Check sheet for the modelled part. Datum: model origin and axes. Units: mm. A direction names the side the tool comes from. Round coordinates to 2 decimals unless told otherwise and drop trailing zeros. Loops run counter-clockwise (first coordinate to the right, second up) from the corner with the lowest first, then second, coordinate; pieces in that order, holes last. Notation, with made-up numbers: (35, -14) -> (91, -14) arc R25 ccw to (91, 3) -> close; hole circle Ø4 at (14, 11). An arc over 180 degrees is marked (long way). One line per question, with ' | ' between items.
Autodesk Inventor part; units mm, degrees
sketch "HeadplateSketch" plane through (0, 0, 0) normal (0, 0, 1) x (1, 0, 0)
  line L0 (22.2193, -2.4109) -> (25.4193, -1.6109)
  line L1 (25.4193, -1.6109) -> (25.4193, -0.0109)
  line L2 (6.3193, 0.7891) -> (3.1193, -0.0109)
  line L3 (3.1193, -1.6109) -> (3.1193, -0.0109)
  line L4 (6.3193, 0.7891) -> (22.2193, 0.7891)
  line L5 (22.2193, 0.7891) -> (25.4193, -0.0109)
  line L6 (17.1922, 9.6958) -> (17.1922, -2.4109)
  line L7 (17.1922, 9.6958) -> (18.128, 9.6958)
  line L8 (17.1922, 9.6958) -> (15.1602, 9.6958)
  line L9 (11.7996, 5.443) -> (11.7996, -2.4109)
  line L10 (21.4383, 5.5008) -> (21.4383, -2.4109)
  line L11 (21.4383, 5.5008) -> (18.128, 9.6958)
  arc A0 (15.1602, 9.6958) -> (11.7996, 5.443) centre (17.4689, 4.4173) ccw
  line L12 (3.1193, -1.6109) -> (6.3193, -2.4109)
  line L13 (6.3193, -2.4109) -> (22.2193, -2.4109)
  point P0 (11.7996, 0.7891)
  dimension "d95" = 3.2
  dimension "d102" = 1.6
  dimension "d104" = 3.2
  dimension "d106" = 0.8
  dimension "d109" = 1.6
  dimension "d110" = 3.2
  dimension "d112" = 22.3
  dimension "d113" = 15.9
extrude "拉伸1" add sketch "HeadplateSketch" along normal blind 1.27
extrude "拉伸8" add sketch "HeadplateSketch" against normal blind 1.5 contours L13 L6 L4 L10 | L4 L6 L7 L11 L10 | L13 L9 L4 L6 | L4 L9 A0 L8 L6
sketch "草图2" plane through (15.1602, 9.6958, 1.27) normal (0, 1, 0) x (1, 0, 0)
  line L0 (-3.3633, 2.0352) -> (1.9994, 0)
  arc A0 (-3.3633, 2.77) -> (6.2787, 1.2693) centre (3.7754, 16.9113) ccw
  line L1 (1.9994, 0) -> (6.2787, 0)
  line L2 (-3.3633, 2.77) -> (6.2787, 2.77)
  line L3 (2.9678, 2.77) -> (0, 2.77)
  line L4 (6.2787, 1.2693) -> (6.2787, 2.77)
  line L5 (-3.3633, 0) -> (1.9994, 0)
  line L6 (0, 0) -> (2.9678, 0)
  line L7 (2.9678, 0) -> (2.9678, 2.77)
  line L8 (-3.3633, 0) -> (-3.3633, 2.0352)
extrude "拉伸4" cut sketch "草图2" against normal up to next contours A0 L2 L7 | L7 L2 L4 A0
sketch "草图6" plane through (6.3193, -2.4109, 0) normal (0, -1, 0) x (1, 0, 0)
  line L0 (0, 0) -> (5.5435, 0)
  line L1 (0.6566, 0) -> (5.5435, -1.4987)
  line L2 (5.5435, 0) -> (5.5435, -1.4987)
  line L3 (0.6566, 0) -> (5.5435, 0)
  arc A0 (15.1197, 0.0007) -> (5.4803, -1.4987) centre (12.6164, -15.6413) ccw
  line L4 (15.1197, 0.0007) -> (15.1197, 0)
  line L5 (15.1197, 0) -> (15.9, 0)
  line L6 (15.9, 0) -> (15.9, 1.27)
  line L7 (15.9, 1.27) -> (0, 1.27)
  line L8 (0, 0) -> (0, 1.27)
  line L9 (0, 0) -> (5.4803, 0)
  line L10 (5.4803, 0) -> (5.4803, -1.4987)
extrude "拉伸7" add sketch "草图6" against normal up to surface (3.2 mm away) contours L0 L10 L1 | L0 L2 A0 L1 L10 | A0 L2 L1
sketch "草图3" plane through (6.3193, 0.7891, 0) normal (0, 1, 0) x (1, 0, 0)
  line L0 (0, -1.27) -> (5.4803, -1.27)
  line L1 (5.4803, 0) -> (5.4803, -1.27)
  line L2 (5.4803, 0) -> (0, 0)
  line L3 (0, 0) -> (0, -1.27)
  line L4 (5.4803, -1.27) -> (16.1538, -1.27)
  line L5 (16.1538, -1.27) -> (17.1139, -1.27)
  line L6 (17.1139, -1.27) -> (17.1139, 0.0011)
extrude "拉伸9" cut sketch "草图2" against normal up to surface (8.9067 mm away) contours L0 L5 L8
sketch "草图4" plane through (0, 0, 1.27) normal (0, 0, 1) x (1, 0, 0)
  circle A0 centre (17.2686, 8.053) radius 0.825
  circle A1 centre (18.9292, 5.4282) radius 0.825
  circle A2 centre (19.0006, 2.5892) radius 0.825
  circle A3 centre (17.1095, -0.097) radius 0.825
  line L0 (6.3193, 0.7891) -> (11.7996, 0.7891)
  line L1 (12.1356, 5.3815) -> (12.1356, 2.0023)
  line L2 (12.1356, 5.3815) -> (17.1561, 5.3815)
  line L3 (17.1561, 5.3815) -> (17.1561, 2.008)
  line L4 (17.1561, 2.008) -> (12.1356, 2.008)
  line L5 (11.7983, 4.0675) -> (12.1356, 4.0675)
  arc A4 (17.1561, 5.3815) -> (12.1356, 5.3815) centre (14.6459, 4.9584) ccw
  arc A5 (12.1356, 2.008) -> (17.1561, 2.008) centre (14.6459, 5.3033) ccw
  circle A6 centre (19.9896, -0.0785) radius 0.825
  circle A7 centre (14.1001, -0.1524) radius 0.825
extrude "拉伸10" cut sketch "草图4" against normal through all contours L2 L3 L4 L1 | A4 L2 | L4 A5
hole "打孔7" at (18.9292, 5.4282, 1.27) at (19.0006, 2.5892, 1.27) at (17.1095, -0.097, 1.27) at (17.2686, 8.053, 1.27) direction (0, 0, -1) diameter 1.65 end through all
hole "打孔8" at (14.1001, -0.1524, 1.27) at (19.9896, -0.0785, 1.27) direction (0, 0, -1) diameter 1.65 end through all
sketch "Sketch8" plane through (0, 0, 0) normal (0, 0, 1) x (1, 0, 0)
  arc A0 (17.1561, 5.3815) -> (12.1356, 5.3815) centre (14.6459, 4.9584) ccw
  arc A1 (12.1356, 2.008) -> (17.1561, 2.008) centre (14.6459, 5.3033) ccw
  line L0 (17.1596, 7.2353) -> (17.1596, 0.7891)
  line L1 (12.1356, 2.008) -> (12.1356, 5.3815)
  line L2 (14.6459, 7.5041) -> (14.6459, 1.1608)
  line L3 (17.1596, 4.3324) -> (12.1356, 4.3324)
  line L4 (-5.0839, 0) -> (30.5031, 0)
  line L5 (0, 12.1209) -> (0, -4.8328)
  point P0 (0, 0)
  dimension "d116" = 6.3433
  dimension "d117" = 3.1717
  dimension "d118" = 14.6459
  dimension "d119" = 4.3324
sketch "Sketch9" plane through (11.7996, 0.7891, -0.7642) normal (-0.3548, 0, 0.9349) x (0.9349, 0, 0.3548)
  ellipse E0 centre (5.8496, 7.2639) end of major axis (6.7321, 7.2639) minor radius 0.825 (5.7331, 8.0816) -> (5.7331, 6.4461) ccw
  line L0 (5.7331, 8.9067) -> (5.7331, 8.0816)
  line L1 (3.5945, 8.9067) -> (5.7331, 8.9067)
  ellipse E1 centre (6.0638, 3.6282) end of major axis (-0.0984, 3.6282) minor radius 5.7613 (3.5945, 8.9067) -> (0, 4.6539) ccw
  line L2 (0, 0) -> (0, 4.6539)
  line L3 (0, 0) -> (5.7331, 0)
  line L4 (5.7331, 6.4461) -> (5.7331, 0)
  line L5 (5.7293, 4.5923) -> (5.7293, 1.2188)
  ellipse E2 centre (3.0444, 4.5141) end of major axis (-1.3864, 4.5141) minor radius 4.1425 (0.3594, 1.2188) -> (5.7293, 1.2188) ccw
  line L6 (0.3594, 1.2188) -> (0.3594, 4.5923)
  ellipse E3 centre (3.0444, 4.1693) end of major axis (5.7672, 4.1693) minor radius 2.5457 (5.7293, 4.5923) -> (0.3594, 4.5923) ccw
  line L7 (5.3145, 1.2188) -> (5.3145, 4.5923)
  arc A0 (0.112, 1.2188) -> (5.3145, 1.2188) centre (5.3145, 1.2188) ccw
  arc A1 (5.3145, 4.5923) -> (0.112, 4.5923) centre (0.112, 4.5923) ccw
  line L8 (5.3145, 4.5923) -> (0.3594, 4.5923)
  line L9 (2.8369, 6.7075) -> (4.6638, 6.7075)
  line L10 (2.8369, 0.3762) -> (5.3145, 0.3762)
  line L11 (2.8369, 6.7075) -> (2.8369, 0.3762)
  line L12 (2.8369, 3.5419) -> (5.3145, 3.5419)
  line L13 (2.9322, 6.7149) -> (2.9322, 0.3716)
  point P0 (-10.7607, -0.7891)
  dimension "d121" = 0.0953
ref_plane "Work Plane3" through (11.7996, 0.7891, -0.7642) normal (-0.3548, 0, 0.9349) x (0.9349, 0, 0.3548)
ref_plane "Work Plane1" through (14.558, 0, 0) normal (1, 0, 0) x (0, 1, 0)
ref_plane "Work Plane2" through (0, 4.332, 0) normal (0, 1, 0) x (-1, 0, 0)
ref_plane "Work Plane4" through (0, 0, 0.283) normal (0, 0, 1) x (1, 0, 0)
sketch "Sketch10" plane through (0, 0, 0) normal (0, 0, 1) x (1, 0, 0)
  line L0 (3.1193, -1.6109) -> (3.1193, -0.0109)
  line L1 (3.1193, -0.8109) -> (0, -0.8109)
  line L2 (25.404, -0.8109) -> (34.4809, -0.8109)
  point P0 (0, 0)
  dimension "d126" = 0.8109
ref_plane "Work Plane5" through (0, -0.811, 0) normal (0, 1, 0) x (-1, 0, 0)
sketch "Sketch11" plane through (11.7996, 0.7891, -0.7642) normal (-0.3548, 0, 0.9349) x (0.9349, 0, 0.3548)
  ellipse E0 centre (5.8496, 7.2639) end of major axis (6.7321, 7.2639) minor radius 0.825 (5.7331, 8.0816) -> (5.7331, 6.4461) ccw
  line L0 (5.7331, 8.9067) -> (5.7331, 8.0816)
  line L1 (3.5945, 8.9067) -> (5.7331, 8.9067)
  ellipse E1 centre (6.0638, 3.6282) end of major axis (-0.0984, 3.6282) minor radius 5.7613 (3.5945, 8.9067) -> (0, 4.6539) ccw
  line L2 (0, 0) -> (0, 4.6539)
  line L3 (0, 0) -> (5.7331, 0)
  line L4 (5.7331, 6.4461) -> (5.7331, 0)
  line L5 (5.7293, 4.5923) -> (5.7293, 1.2188)
  ellipse E2 centre (3.0444, 4.5141) end of major axis (-1.3864, 4.5141) minor radius 4.1425 (0.3594, 1.2188) -> (5.7293, 1.2188) ccw
  line L6 (0.3594, 1.2188) -> (0.3594, 4.5923)
  ellipse E3 centre (3.0444, 4.1693) end of major axis (5.7672, 4.1693) minor radius 2.5457 (5.7293, 4.5923) -> (0.3594, 4.5923) ccw
  circle A0 centre (3.0444, 3.5307) radius 3.5
  point P0 (-10.7607, -0.7891)
  dimension "d128" = 7
ref_plane "Work Plane6" through (12.0474, 0.7891, -1.4172) normal (-0.3548, 0, 0.9349) x (0.9349, 0, 0.3548)
sketch "Sketch12" plane through (0, 0, 1.27) normal (0, 0, 1) x (1, 0, 0)
  circle A0 centre (17.1095, -0.097) radius 0.825
  line L0 (14.541, 7.5041) -> (14.541, 1.1608)
  point P0 (0, 0)
  dimension "d130" = 2.5684
equation "\"d117\" = 0.5 * d116"
properties part number "MPS Headpost" material "Titanium"
(1) Mould release check, pull along X, two halves, no side actions. Record for faces 1 (the face through (3.119, -1, 1)), 2 (the face through (10, 0.789, 0)), 3 (the face through (13.28, -0.05, 0.43)): +X half, -X half, draft (parallel to the pull), parting line (faces both ways), or undercut.
Answer:
face 1: -X half | face 2: draft | face 3: undercut
(2) Go/stop test with flat-tipped pins: pin 1 (1 mm diameter, centred on y = 5.5, z = -1, fed in from +X); pin 2 (1.3 mm diameter, centred on x = 19, y = 2.59, fed in from +Z); pin 3 (2.5 mm diameter, centred on x = 24, y = -1, fed in from -Z); pin 4 (1 mm diameter, centred on y = 8, z = 0, fed in from +X). Record where each tip stops, or that it passes through.
Answer:
pin 1: stops at x = 12.32 | pin 2: passes through | pin 3: stops at z = 0 | pin 4: stops at x = 19.84
(3) Scan lines: probe 1 along X at (y, z) = (4.75, 1.2); probe 2 along X at (y, z) = (2.25, 0.55); probe 3 along Z at (x, y) = (21.5, 0.5). Record each from-to range of solid material in increasing order.
Answer:
probe 1: x = 17.16 to 18.46, 19.4 to 21.44 | probe 2: x = 17.16 to 18.25, 19.75 to 21.44 | probe 3: z = 0 to 1.27
(4) Sectioned sample at C-C, the plane y = -0.5. Count the separate pieces of the cut face and the enclosed holes in it, and give its area (3 significant figures).
Answer:
separate pieces: 4 | enclosed holes: 0 | area: 28.1 mm2
(5) Set-up check for faces 4 (the face through (17.156, 4, 1)), 5 (the face through (21.438, 3, 1)), 6 (the face through (15.03, 1.18, -0.03)), 7 (the face through (5, -1, 0)): record each of +Z, -Z, +X, -X, +Y, -Y from which the full face is reachable in a straight line by a thin tool's end or side.
Answer:
face 4: +Z, -Z, -X | face 5: +Z, -Z, +X, +Y | face 6: +Z, -Z | face 7: -Z, -X, +Y, -Y
(6) Sectioned sample at A-A, the plane x = 13. Record the cut outline in (y, z).
Answer:
outline: (-2.41, -0.95) -> (1.5, -0.95) -> (1.5, -0.31) -> (0.79, -0.31) -> (0.79, 1.27) -> (-2.41, 1.27) -> close; (6.9, -0.95) -> (8.05, -0.95) -> (8.05, -0.31) -> (6.9, -0.31) -> close
